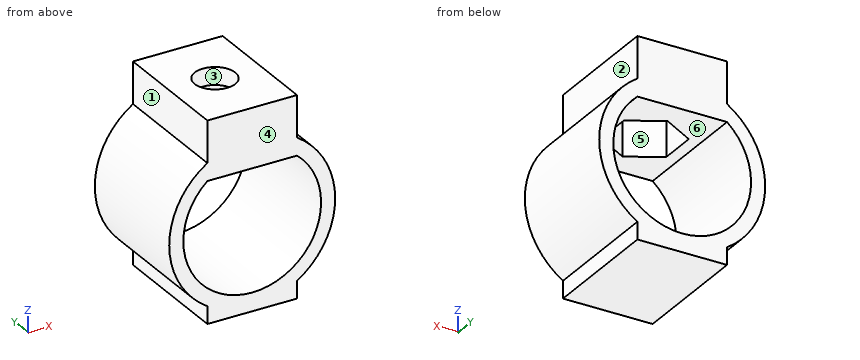
```python
from build123d import *

# Parameters (mm, degrees)
PAD002_DEPTH    = 15
POCKET_DEPTH    = 5
SKETCH007_R     = 2.45
POCKET001_DEPTH = 2.115274
PAD003_DEPTH    = 15


with BuildPart() as part:
    # Sketch002 (on DatumPlane) → Pad002 (new body)
    with BuildSketch(Plane.XZ.offset(20)):
        with BuildLine():
            ThreePointArc((-5.403702, 8.414274), (0, -10), (5.403702, 8.414274))
            Line((5.403702, 13.414274), (5.403702, 8.414274))
            Line((-5.403702, 13.414274), (5.403702, 13.414274))
            Line((-5.403702, 8.414274), (-5.403702, 13.414274))
        make_face()
        with BuildLine():
            ThreePointArc((-5.403702, 6.3), (0, -8.3), (5.403702, 6.3))
            Line((-5.403702, 6.3), (5.403702, 6.3))
        make_face(mode=Mode.SUBTRACT)
    extrude(amount=PAD002_DEPTH)

    # Sketch006 (on Face6 of Pad002) → Pocket (cut)
    with BuildSketch(Plane(origin=(0, -20, 6.3), x_dir=(1, 0, 0), z_dir=(0, 0, -1))):
        Polygon((-3.925, 9.7661), (-3.925, 5.2339), (0, 2.9678), (3.925, 5.2339), (3.925, 9.7661), (0, 12.0322), align=None)
    extrude(amount=-POCKET_DEPTH, mode=Mode.SUBTRACT)

    # Sketch007 (on Face15 of Pocket) → Pocket001 (cut, through all)
    with BuildSketch(Plane(origin=(0, -20, 11.3), x_dir=(1, 0, 0), z_dir=(0, 0, -1))):
        with Locations((0, 7.5)):
            Circle(SKETCH007_R)
    extrude(amount=-POCKET001_DEPTH, mode=Mode.SUBTRACT)

    # Sketch008 (on Face5 of Pocket001) → Pad003 (join)
    with BuildSketch(Plane.XZ.offset(35)):
        with BuildLine():
            Line((-5.403702, -8.414274), (-5.403702, -10.5))
            Line((-5.403702, -10.5), (5.403702, -10.5))
            Line((5.403702, -10.5), (5.403702, -8.414274))
            ThreePointArc((-5.403702, -8.414274), (0, -10), (5.403702, -8.414274))
        make_face()
    extrude(amount=-PAD003_DEPTH)


solid = part.part
```
Input: part model. Units: mm. Frame: model coordinates. Face numbers are marked on the shaded views. A direction names the side the tool comes from. Give positions to 0.01 mm unless a question says otherwise; leave off trailing zeros. Order: outer loops, then holes, each group sorted by start corner. A loop starts at its lowest first (then second) coordinate and runs counter-clockwise, first axis right, second up. Notation, with made-up numbers: (-16, 58.5) - (-6, 58.5) arc R28 ccw to (-6, 93.5) - close; hole circle Ø3 at (12, 11.25). An arc over 180 degrees is marked (long way). Use a Markdown table: item, result.
(1) Line query: line 1 (X direction, y = -30.75, z = 0); line 2 (Z direction, x = 0, y = -31); line 3 (Z direction, x = 0, y = -32.5). Output: solid intervals per line, ascending. Write a range as from..to.
Computed values:
| item | result |
|---|---|
| line 1 | x = -10..-8.3, 8.3..10 |
| line 2 | z = -10.5..-8.3, 11.3..13.41 |
| line 3 | z = -10.5..-8.3, 6.3..13.41 |
(2) Draft query along Y for the marked faces 4, 5 and 6. Return one class per face: released by +Y, released by -Y, zero draft, split by the parting line, or undercut.
Computed values:
| item | result |
|---|---|
| face 4 | released by -Y |
| face 5 | undercut |
| face 6 | zero draft |
(3) Section query B-B (y = -27.5). Output: boundary loops of the cut face in (x, z) (3 decimals).
Computed values:
| item | result |
|---|---|
| outline | (-5.404, -10.5) - (5.404, -10.5) - (5.404, -8.414) arc R10 ccw to (5.404, 8.414) - (5.404, 13.414) - (2.45, 13.414) - (2.45, 11.3) - (3.925, 11.3) - (3.925, 6.3) - (5.404, 6.3) arc R8.3 cw (long way) to (-5.404, 6.3) - (-3.925, 6.3) - (-3.925, 11.3) - (-2.45, 11.3) - (-2.45, 13.414) - (-5.404, 13.414) - (-5.404, 8.414) arc R10 ccw to (-5.404, -8.414) - close |
(4) Section query C-C (y = -31.25). Output: boundary loops of the cut face in (x, z).
Computed values:
| item | result |
|---|---|
| outline | (-5.4, -10.5) - (5.4, -10.5) - (5.4, -8.41) arc R10 ccw to (5.4, 8.41) - (5.4, 13.41) - (-5.4, 13.41) - (-5.4, 8.41) arc R10 ccw to (-5.4, -8.41) - close; hole (-5.4, 6.3) arc R8.3 ccw (long way) to (5.4, 6.3) - (1.35, 6.3) - (1.35, 11.3) - (-1.35, 11.3) - (-1.35, 6.3) - close |
(5) Access query for the marked faces 1, 2 and 3. Directions: +Z, -Z, +X, -X, +Y, -Y. A direction counts if a zero-diameter tool reaches every point of the face in a straight line with its end or side. Return the directions, or none.
Computed values:
| item | result |
|---|---|
| face 1 | +Z, -X, +Y, -Y |
| face 2 | +Z, +X, +Y, -Y |
| face 3 | +Z |
(6) Section query D-D (x = -3.5). Output: boundary loops of the cut face in (y, z), then the cut area to 3 significant figures.
Computed values:
| item | result |
|---|---|
| outline | (-35, -10.5) - (-20, -10.5) - (-20, -7.53) - (-35, -7.53) - close; (-35, 6.3) - (-30.01, 6.3) - (-30.01, 11.3) - (-24.99, 11.3) - (-24.99, 6.3) - (-20, 6.3) - (-20, 13.41) - (-35, 13.41) - close |
| area | 126 mm2 |
(7) Pin query (flat end, axial travel): pin 1 (10 mm diameter, centred on x = 0, z = 0, fed in from +Y); pin 2 (2.5 mm diameter, centred on y = -28, z = 8.5, fed in from -X); pin 3 (2.5 mm diameter, centred on y = -24, z = 10.5, fed in from +X); pin 4 (4 mm diameter, centred on y = -24, z = 10, fed in from -X). Return the tip coordinate at first contact, or that it passes through.
Computed values:
| item | result |
|---|---|
| pin 1 | passes through |
| pin 2 | stops at x = -6.89 |
| pin 3 | stops at x = 5.4 |
| pin 4 | stops at x = -6 |
(8) Section query A-A (z = 0). Output: boundary loops of the cut face in (x, y), then the cut area to 3 significant figures.
Computed values:
| item | result |
|---|---|
| outline | (-10, -35) - (-8.3, -35) - (-8.3, -20) - (-10, -20) - close; (8.3, -35) - (10, -35) - (10, -20) - (8.3, -20) - close |
| area | 51.0 mm2 |
